Work out the finished part from the listing and answer in its coordinate system (mm). A direction names the side the tool comes from. Give positions to 0.01 mm unless a question says otherwise; leave off trailing zeros. Loops run counter-clockwise (first coordinate to the right, second up) from the corner with the lowest first, then second, coordinate; pieces in that order, holes last. Notation, with made-up numbers: (66, 39) - (96, 39) arc R24 cw to (96, 62) - close; hole circle Ø9 at (-24.5, 53.25). An arc over 180 degrees is marked (long way). One line per item, written item: value.
from build123d import *

# Parameters (mm, degrees)
BASPROSKE_W        = 10
BASPROSKE_H        = 12.5
TOOTHCUT_DEPTH     = 21.310096012
TEETHCUTS_COUNT    = 18
TEETHCUTS_ANGLE    = 340
BORSKE_R           = 1.5
BORE_DEPTH         = 50.0000508
SKETCH1_R          = 8.5
CUT_EXTRUDE1_DEPTH = 6
SKETCH2_R          = 3.2
CUT_EXTRUDE2_DEPTH = 19.575045867


with BuildPart() as part:
    # BasProSke → Base-Revolve (revolve)
    with BuildSketch(Plane(origin=(0, 0, 0), x_dir=(1, 0, 0), z_dir=(0, 1, 0)), mode=Mode.PRIVATE) as base_revolve_sk:
        with Locations((5, 6.25)):
            Rectangle(BASPROSKE_W, BASPROSKE_H)
    revolve(base_revolve_sk.sketch.rotate(Axis((-10, 0, 0), (1, 0, 0)), 180), axis=Axis((-10, 0, 0), (1, 0, 0)))

    # TooCutSke → ToothCut (cut, through all)
    with BuildSketch(Plane(origin=(0, 0, 0), x_dir=(0, 0, -1), z_dir=(1, 0, 0))):
        with BuildLine():
            ThreePointArc((0.634554124, 9.665693111), (0, 9.6865), (-0.634554124, 9.665693111))
            ThreePointArc((-0.634554124, 9.665693111), (-1.026818848, 11.131124412), (-1.883745888, 12.38293772))
            ThreePointArc((-1.883745888, 12.38293772), (0, 12.5254), (1.883745888, 12.38293772))
            ThreePointArc((1.883745888, 12.38293772), (1.026818848, 11.131124412), (0.634554124, 9.665693111))
        make_face()
    toothcut = extrude(amount=TOOTHCUT_DEPTH, mode=Mode.SUBTRACT)

    # TeethCuts: ToothCut ×18 about axis
    teethcuts_axis = Axis((-10, 0, 0), (1, 0, 0))
    for i in range(1, TEETHCUTS_COUNT):
        add(toothcut.rotate(teethcuts_axis, i * TEETHCUTS_ANGLE / (TEETHCUTS_COUNT - 1)), mode=Mode.SUBTRACT)

    # BorSke → Bore (cut, symmetric)
    with BuildSketch(Plane(origin=(0, 0, 0), x_dir=(0, 0, -1), z_dir=(1, 0, 0))):
        with Locations(Location((0, 0, 0), (0, 0, 180))):
            Circle(BORSKE_R)
    extrude(amount=BORE_DEPTH, both=True, mode=Mode.SUBTRACT)

    # Sketch1 → Cut-Extrude1 (cut)
    with BuildSketch(Plane(origin=(10, 0, 0), x_dir=(0, 0, -1), z_dir=(1, 0, 0))):
        Circle(SKETCH1_R)
    extrude(amount=-CUT_EXTRUDE1_DEPTH, mode=Mode.SUBTRACT)

    # Sketch2 → Cut-Extrude2 (cut, through all)
    with BuildSketch(Plane(origin=(4, 0, 0), x_dir=(0, 0, -1), z_dir=(1, 0, 0))):
        Circle(SKETCH2_R)
    extrude(amount=-CUT_EXTRUDE2_DEPTH, mode=Mode.SUBTRACT)


solid = part.part
1. Find the intervals of material crossed by line 1 along Y through (x, z) = (5.55, 0); line 2 along Y through (x, z) = (1.7, 0); line 3 along Z through (x, y) = (5, -9.5), in increasing order.
Output:
line 1: y = -9.69 to -8.5, 8.5 to 9.69
line 2: y = -9.69 to -3.2, 3.2 to 9.69
line 3: z = -6.44 to -4.27, -2.76 to 2.76, 4.27 to 6.44
2. For faces 4 (the cylindrical face through (4.93, 10.113, -4.776)), 5 (the cylindrical face through (4.93, 7.415, -6.233)), 6 (the cylindrical face through (4.93, -7.87, 7.95)), determine the directions among +Z, -Z, +X, -X, +Y, -Y from which every point of the face is accessible in a straight line to the end or side of a thin tool.
Output:
face 4: +X, -X, +Y
face 5: +X, -X
face 6: +X, -X, -Y
3. Section C-C (z = 4.75) is taken. Write down the section's boundary in (x, y).
Output:
outline: (0, -10.09) - (10, -10.09) - (10, -7.05) - (4, -7.05) - (4, 7.05) - (10, 7.05) - (10, 10.09) - (0, 10.09) - close
4. Section D-D (y = -6.25) is taken. Write down the section's boundary in (x, z).
Output:
outline: (0, -8.97) - (10, -8.97) - (10, -5.76) - (4, -5.76) - (4, 5.76) - (10, 5.76) - (10, 8.97) - (0, 8.97) - close
5. The mould has two halves that part along Z. Classify faces 1 (the cylindrical face through (4.93, 2.92, -10.75)), 2 (the cylindrical face through (4.93, -10.774, 2.845)), 3 (the flat face through (0, 3, 3)): released by +Z, released by -Z, zero draft, split by the parting line, or undercut.
Output:
face 1: released by -Z
face 2: undercut
face 3: zero draft
6. Flat-ended cylindrical pins translate along their axes: pin 1 Ø5 at (x, y) = (4, 4) entering from +Z; pin 2 Ø5 at (y, z) = (-3.5, -1.5) entering from +X; pin 3 Ø1.5 at (x, z) = (4, 6) entering from -Y; pin 4 Ø4 at (y, z) = (0, 0) entering from -X. Find the tip coordinate at first contact, or state that the pin passes through.
Output:
pin 1: stops at z = 11.85
pin 2: stops at x = 4
pin 3: stops at y = -10.98
pin 4: passes through
7. Section B-B (y = 0) is taken. Write down the section's boundary in (x, z).
Output:
outline: (0, -12.5) - (10, -12.5) - (10, -8.5) - (4, -8.5) - (4, -3.2) - (0, -3.2) - close; (0, 3.2) - (4, 3.2) - (4, 8.5) - (10, 8.5) - (10, 12.5) - (0, 12.5) - close
8. Section A-A (z = 0) is taken. Write down the section's boundary in (x, y), and give its area (3 significant figures).
Output:
outline: (0, -9.69) - (10, -9.69) - (10, -8.5) - (4, -8.5) - (4, -3.2) - (0, -3.2) - close; (0, 3.2) - (4, 3.2) - (4, 8.5) - (10, 8.5) - (10, 9.69) - (0, 9.69) - close
area: 66.1 mm²
